The listing builds one solid part. Answer for the finished solid, in the listing's coordinates (mm). Face numbers are marked on the shaded views. Round coordinates to 2 decimals unless told otherwise and drop trailing zeros. Write each loop counter-clockwise with the first axis right and the second up, starting at its lowest first coordinate (ties: lowest second). Pieces come first, ordered by that corner, then holes.
Item 1: Find section C-C on y = 16.5. Give the vertices of the cut face in (x, z), then the cut area to 3 significant figures.
Item 2: Find section A-A on x = 17. Give the vertices of the cut face in (y, z).
Item 3: Each of these flat-tipped pins is pushed along its axis until it touches: pin 1 (8 mm diameter, centred on x = 34.5, y = 10.5, fed in from -Z); pin 2 (2.5 mm diameter, centred on x = 33.75, z = 28.83, fed in from +Y); pin 3 (3 mm diameter, centred on x = 52.5, y = -22.1, fed in from +Z). Where does it stop, or does it pass through?
Item 4: Find the intervals of material crossed by probe 1 along Z at (x, y) = (24.25, -33); probe 2 along Z at (x, y) = (49, -4); probe 3 along Z at (x, y) = (38.5, -33.8), in increasing order.
Item 5: For a pull along Z with two mould halves and no side action, classify the marked faces 1, 2 and 3 as +Z half, -Z half, draft (parallel to the pull), parting line (faces both ways), or undercut.
Item 6: Find section D-D on z = -14.5. Give the vertices of the cut face in (x, y).
Item 7: Find section B-B on x = 5.5. Give the vertices of the cut face in (y, z), then the cut area to 3 significant figures.
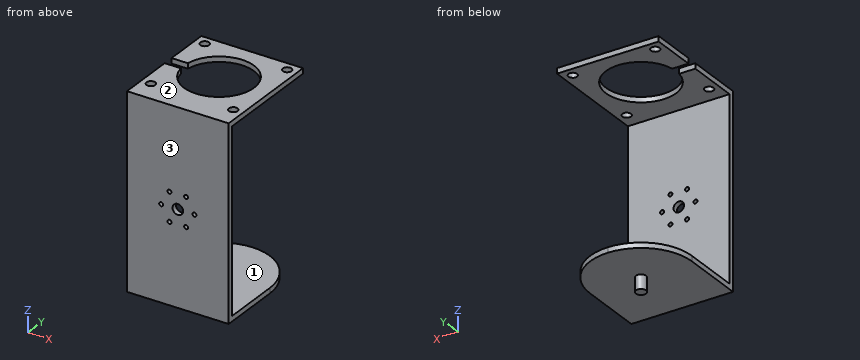
```python
from build123d import *

# Parameters (mm, degrees)
BOSS_EXTRUDE1_DEPTH       = 58
SKETCH2_R                 = 2.5
SKETCH2_R_2               = 20
CUT_EXTRUDE1_DEPTH        = 58
CUT_EXTRUDE2_DEPTH        = 58
CUT_EXTRUDE3_DEPTH        = 58
SKETCH5_R                 = 2.95
BOSS_EXTRUDE2_DEPTH       = 8
SKETCH7_W                 = 29
SKETCH7_H                 = 6
CUT_EXTRUDE5_DEPTH        = 10
F_4_40_TAPPED_HOLE4_D     = 2.2606
F_4_40_TAPPED_HOLE4_DEPTH = 7.6
F_4_40_TAPPED_HOLE4_TIP   = 0.679152758
SKETCH25_R                = 3
CUT_EXTRUDE6_DEPTH        = 10
SKETCH26_W                = 103.5
SKETCH26_H                = 2
CUT_EXTRUDE7_DEPTH        = 90


with BuildPart() as part:
    # Sketch1 → Boss-Extrude1 (new body)
    with BuildSketch(Plane(origin=(0, 0, 0), x_dir=(0, 0, -1), z_dir=(1, 0, 0))):
        Polygon((-73.351671883, 30.400809615), (-73.351671883, -29.599190385), (30.148328117, -29.599190385), (30.148328117, 30.400809615), (33.148328117, 30.400809615), (33.148328117, -34.599190385), (-76.351671883, -34.599190385), (-76.351671883, 30.400809615), align=None)
    extrude(amount=BOSS_EXTRUDE1_DEPTH)

    # Sketch2 → Cut-Extrude1 (cut)
    with BuildSketch(Plane.XY.offset(76.351671883)):
        with Locations((5.5, 24.900809615)):
            Circle(SKETCH2_R)
        with Locations((52.5, 24.900809615)):
            Circle(SKETCH2_R)
        with Locations((52.5, -22.099190385)):
            Circle(SKETCH2_R)
        with Locations((5.5, -22.099190385)):
            Circle(SKETCH2_R)
        with Locations((29, 1.400809615)):
            Circle(SKETCH2_R_2)
    extrude(amount=-CUT_EXTRUDE1_DEPTH, mode=Mode.SUBTRACT)

    # Sketch3 → Cut-Extrude2 (cut)
    with BuildSketch(Plane(origin=(0, 0, -33.148328117), x_dir=(-1, 0, 0), z_dir=(0, 0, -1))):
        with BuildLine():
            Line((-29, 30.400809615), (-58, 30.400809615))
            Line((-58, 30.400809615), (-58, 1.400809615))
            ThreePointArc((-58, 1.400809615), (-49.506096654, 21.90690627), (-29, 30.400809615))
        make_face()
    extrude(amount=-CUT_EXTRUDE2_DEPTH, mode=Mode.SUBTRACT)

    # Sketch4 → Cut-Extrude3 (cut)
    with BuildSketch(Plane(origin=(0, 0, -33.148328117), x_dir=(-1, 0, 0), z_dir=(0, 0, -1))):
        with BuildLine():
            Line((-29, 30.400809615), (0, 30.400809615))
            Line((0, 30.400809615), (0, 1.400809615))
            ThreePointArc((0, 1.400809615), (-8.493903346, 21.90690627), (-29, 30.400809615))
        make_face()
    extrude(amount=-CUT_EXTRUDE3_DEPTH, mode=Mode.SUBTRACT)

    # Sketch5 → Boss-Extrude2 (add)
    with BuildSketch(Plane(origin=(0, 0, -33.148328117), x_dir=(-1, 0, 0), z_dir=(0, 0, -1))):
        with Locations((-29, 1.400809615)):
            Circle(SKETCH5_R)
    extrude(amount=BOSS_EXTRUDE2_DEPTH)

    # Sketch7 → Cut-Extrude5 (cut)
    with BuildSketch(Plane.XY.offset(76.351671883)):
        with Locations((14.5, 1.400809615)):
            Rectangle(SKETCH7_W, SKETCH7_H)
    extrude(amount=-CUT_EXTRUDE5_DEPTH, mode=Mode.SUBTRACT)

    # #4-40 Tapped Hole4
    with Locations(Plane(origin=(0, -34.599190385, 0), x_dir=(-1, 0, 0), z_dir=(0, -1, 0))):
        with Locations((-19.5, -20.601671883), (-24.25, -28.828913219), (-33.75, -28.828913219), (-38.5, -20.601671883), (-33.75, -12.374430547), (-24.25, -12.374430547)):
            Hole(F_4_40_TAPPED_HOLE4_D / 2, depth=F_4_40_TAPPED_HOLE4_DEPTH)
            with Locations((0, 0, -(F_4_40_TAPPED_HOLE4_DEPTH + F_4_40_TAPPED_HOLE4_TIP / 2))):  # 118° drill point
                Cone(0, F_4_40_TAPPED_HOLE4_D / 2, F_4_40_TAPPED_HOLE4_TIP, mode=Mode.SUBTRACT)

    # Sketch25 → Cut-Extrude6 (cut)
    with BuildSketch(Plane.XZ.offset(34.599190385)):
        with Locations((29, 20.601671883)):
            Circle(SKETCH25_R)
    extrude(amount=-CUT_EXTRUDE6_DEPTH, mode=Mode.SUBTRACT)

    # Sketch26 → Cut-Extrude7 (cut)
    with BuildSketch(Plane(origin=(58, 0, 0), x_dir=(0, 0, -1), z_dir=(1, 0, 0))):
        with Locations((-21.601671883, -30.599190385)):
            Rectangle(SKETCH26_W, SKETCH26_H)
    extrude(amount=-CUT_EXTRUDE7_DEPTH, mode=Mode.SUBTRACT)


solid = part.part
```
Check values:
1. outline: (0, 73.35) - (15.88, 73.35) - (15.88, 76.35) - (0, 76.35) - close; (4.24, -33.15) - (53.76, -33.15) - (53.76, -30.15) - (4.24, -30.15) - close; (42.12, 73.35) - (58, 73.35) - (58, 76.35) - (42.12, 76.35) - close
1. area: 244 mm2
2. outline: (-34.6, -33.15) - (27.8, -33.15) - (27.8, -30.15) - (-31.6, -30.15) - (-31.6, 73.35) - (-14.6, 73.35) - (-14.6, 76.35) - (-34.6, 76.35) - close; (17.4, 73.35) - (30.4, 73.35) - (30.4, 76.35) - (17.4, 76.35) - close
3. pin 1: stops at z = -33.15
3. pin 2: stops at y = -31.6
3. pin 3: stops at z = -30.15
4. probe 1: z = -33.15 to 11.24, 13.5 to 27.7, 29.96 to 76.35
4. probe 2: z = -33.15 to -30.15, 73.35 to 76.35
4. probe 3: z = -33.15 to 19.47, 21.73 to 76.35
5. face 1: undercut
5. face 2: +Z half
5. face 3: draft
6. outline: (0, -34.6) - (58, -34.6) - (58, -31.6) - (0, -31.6) - close
7. outline: (-34.6, -33.15) - (18.39, -33.15) - (18.39, -30.15) - (-31.6, -30.15) - (-31.6, 73.35) - (-24.6, 73.35) - (-24.6, 76.35) - (-34.6, 76.35) - close; (-19.6, 73.35) - (-1.6, 73.35) - (-1.6, 76.35) - (-19.6, 76.35) - close; (4.4, 73.35) - (22.4, 73.35) - (22.4, 76.35) - (4.4, 76.35) - close; (27.4, 73.35) - (30.4, 73.35) - (30.4, 76.35) - (27.4, 76.35) - close
7. area: 616 mm2
